Can you work these out from the model? Positions are in its coordinate system, mm. A direction names the side the tool comes from. Give positions to 0.01 mm unless a question says otherwise; leave off trailing zeros. Order: outer loops, then holes, each group sorted by start corner. A loop starts at its lowest first (then second) coordinate and runs counter-clockwise, first axis right, second up. Notation, with made-up numbers: (-20.5, -12) - (-14.5, -12) arc R18 ccw to (-14.5, 21) - close; hole circle Ø4 at (18, -4). An arc over 180 degrees is marked (long way). Use one line per item in the form item = value. Start each with the question number.
1) Which directions (+Z, -Z, +X, -X, +Y, -Y) give clear straight access to the entire face, cutting with the end or side of a thin tool? Please do faces 1 (the flat face through (44.06, -34.22, 5.01)), 2 (the flat face through (9.525, 14, 5)), 3 (the flat face through (41.365, -28.277, 5.009)), 4 (the flat face through (30.257, -17.458, 5.009)).
2) Suppose I cut it at B-B, the plane y = 13. Write out the boundary of the cut face in (x, z) (3 decimals).
3) Suppose I cut it at A-A, the plane z = 1.25. Write out the boundary of the cut face in (x, y) (1 decimal), and give its area (3 significant figures).
4) For pin 1 (1 mm diameter, centred on y = 10, z = 3.5, fed in from -X); pin 2 (5 mm diameter, centred on x = 25, z = 2.5, fed in from +Y) (3 decimals); pin 3 (5 mm diameter, centred on y = -28.5, z = 5.5, fed in from -X); pin 4 (4 mm diameter, centred on y = -5, z = 7.5, fed in from -X), each with a flat end and sliding along its axis, tell me the tip position at first contact or that it passes through.
5) We'd pull the mould along Y, two halves only. Please class faces 5 (the flat face through (28, 9.525, 5)), 6 (the flat face through (42.6, -8.6, 5)), 7 (the flat face through (0, 9, 5)), 8 (the flat face through (18, 0, 5)): released by +Y, released by -Y, zero draft, split by the parting line, or undercut.
6) Please list where these lines run through material, in increasing order: probe 1 along Y at (x, z) = (16.5, 6.25) (3 decimals); probe 2 along Y at (x, z) = (6.5, 7.75).
Autodesk Inventor part; units mm, degrees
ref_plane "YZ Plane" through (0, 0, 0) normal (1, 0, 0) x (0, 1, 0)
ref_plane "XZ Plane" through (0, 0, 0) normal (0, 1, 0) x (-1, 0, 0)
ref_plane "XY Plane" through (0, 0, 0) normal (0, 0, 1) x (1, 0, 0)
sketch "Sketch1" plane through (0, 0, 0) normal (0, 0, 1) x (1, 0, 0)
  line L0 (0, 0) -> (0, 17.78)
  line L1 (0, 17.78) -> (9.525, 17.78)
  line L2 (9.525, 17.78) -> (9.525, 9.525)
  line L3 (9.525, 9.525) -> (47.625, 9.525)
  line L4 (47.625, 9.525) -> (37.4432, -27.1893)
  line L5 (37.4432, -27.1893) -> (45.398, -29.3954)
  line L6 (45.398, -29.3954) -> (42.6828, -39.1859)
  line L7 (42.6828, -39.1859) -> (25.5495, -34.4344)
  line L8 (25.5495, -34.4344) -> (35.099, 0)
  line L9 (35.099, 0) -> (0, 0)
  dimension "d7" = 17.78
  dimension "d8" = 9.525
  dimension "d9" = 8.255
  dimension "d10" = 38.1
  dimension "d11" = 38.1
  dimension "d12" = 74.5
  dimension "d13" = 8.255
  dimension "d14" = 10.16
  dimension "d15" = 17.78
extrude "Extrusion1" add sketch "Sketch1" along normal blind 10.16
properties part number "AcutePlateAttacher_v1"
Result sheet:
q1.face_1 = +Z, -Z, +X, -Y
q1.face_2 = +Z, -Z, +X, +Y
q1.face_3 = +Z, -Z, +X
q1.face_4 = +Z, -Z, -X
q2.outline = (0, 0) - (9.525, 0) - (9.525, 10.16) - (0, 10.16) - close
q3.outline = (0, 0) - (35.1, 0) - (25.5, -34.4) - (42.7, -39.2) - (45.4, -29.4) - (37.4, -27.2) - (47.6, 9.5) - (9.5, 9.5) - (9.5, 17.8) - (0, 17.8) - close
q3.area = 956 mm²
q4.pin_1 = 0
q4.pin_2 = 9.525
q4.pin_3 = 26.5
q4.pin_4 = 33.16
q5.face_5 = released by +Y
q5.face_6 = undercut
q5.face_7 = zero draft
q5.face_8 = undercut
q6.probe_1 = 0 to 9.525
q6.probe_2 = 0 to 17.78
